The drawing under review shows one solid part. Ordinate dimensions are in mm from its lowest x, y, z. Coordinates: 2 decimals unless noted, no trailing zeros. Write each loop counter-clockwise with the first axis right and the second up, starting at its lowest first coordinate (ties: lowest second). Pieces come first, ordered by that corner, then holes.
Q1. Take a section at C-C (y = 17.5). Give the boundary of the cut face in (x, z), and give its area (3 significant figures).
Q2. For probe 1 along X at (y, z) = (9, 6); probe 2 along Z at (x, y) = (58, 14.75); probe 3 along Z at (x, y) = (60, 11.75), list the stretches that pass through material, from the lowest coordinate up.
Q3. Insertion check: pin 1 (7 mm diameter, centred on x = 82, z = 46, fed in from -Y). The pin has a flat end and moves straight along its axis. Give the tip position at first contact, or say it passes through.
Q4. Take a section at A-A (x = 82). Give the boundary of the cut face in (y, z).
Q5. Take a section at B-B (z = 46). Give the boundary of the cut face in (x, y).
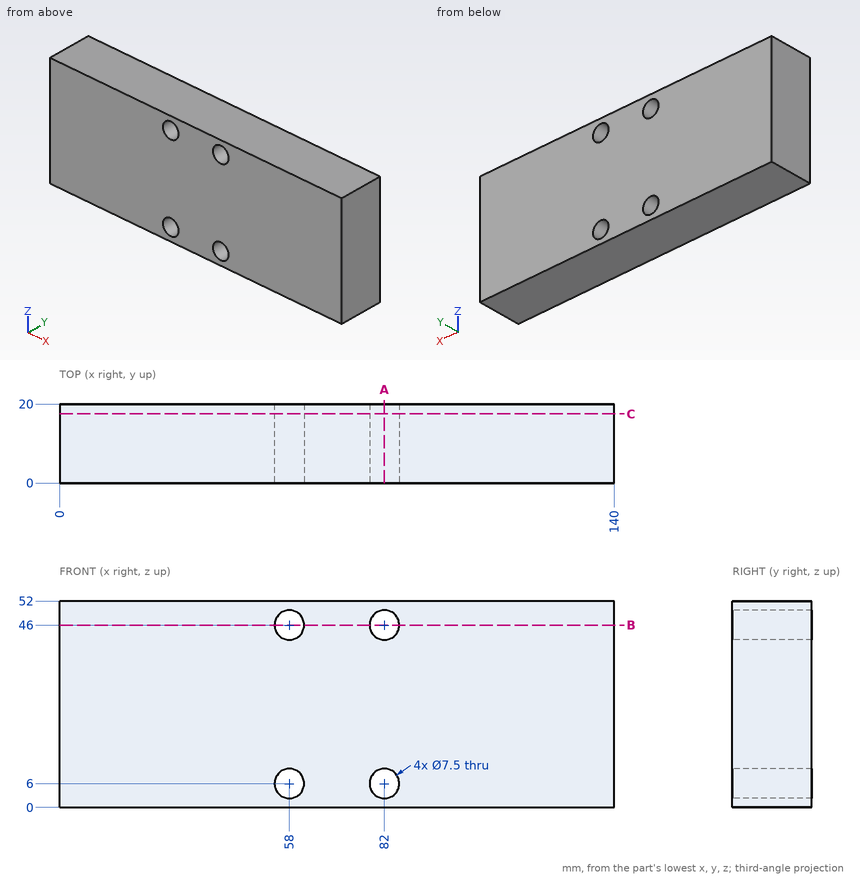
Response:
1. outline: (0, 0) - (140, 0) - (140, 52) - (0, 52) - close; hole circle Ø7.5 at (58, 6); hole circle Ø7.5 at (58, 46); hole circle Ø7.5 at (82, 6); hole circle Ø7.5 at (82, 46)
1. area: 7,100 mm2
2. probe 1: x = 0 to 54.25, 61.75 to 78.25, 85.75 to 140
2. probe 2: z = 0 to 2.25, 9.75 to 42.25, 49.75 to 52
2. probe 3: z = 0 to 2.83, 9.17 to 42.83, 49.17 to 52
3. pin 1: passes through
4. outline: (0, 0) - (20, 0) - (20, 2.25) - (0, 2.25) - close; (0, 9.75) - (20, 9.75) - (20, 42.25) - (0, 42.25) - close; (0, 49.75) - (20, 49.75) - (20, 52) - (0, 52) - close
5. outline: (0, 0) - (54.25, 0) - (54.25, 20) - (0, 20) - close; (61.75, 0) - (78.25, 0) - (78.25, 20) - (61.75, 20) - close; (85.75, 0) - (140, 0) - (140, 20) - (85.75, 20) - close
